For this review, take the finished solid that the model builds, in its own axes (mm). A direction names the side the tool comes from. Coordinates: 2 decimals unless noted, no trailing zeros. Order: outer loops, then holes, each group sorted by start corner. A loop starts at its lowest first (then second) coordinate and runs counter-clockwise, first axis right, second up. Notation, with made-up numbers: M 43,23.5 L 47,23.5 A18 ccw 47,35.5 Z; hole C 4,81 d5. An arc over 180 degrees is marked long. Use one line per item in the form item = value. Start each with the question number.
```python
from build123d import *

# Parameters (mm, degrees)
SKETCH_1_W          = 28
SKETCH_1_H          = 16
EXTRUDE_1_DEPTH     = 5.25
FILLET_1_R          = 3
CUT_EXTRUDE_1_REACH = 21.242
SKETCH_2_R          = 1.5
SKETCH_3_W          = 8.6
SKETCH_3_H          = 6.2
EXTRUDE_2_DEPTH     = 3.4
CUT_EXTRUDE_2_REACH = 21.892
SKETCH_4_W          = 7.6
SKETCH_4_H          = 2.4
SKETCH_5_W          = 8.88
SKETCH_5_H          = 1
EXTRUDE_3_DEPTH     = 3
SKETCH_6_W          = 2.8
SKETCH_6_H          = 4.2
EXTRUDE_4_DEPTH     = 3
FILLET_2_R          = 1.2
EXTRUDE_2_2_DEPTH   = 1.5
SKETCH_7_3_R        = 2.4
EXTRUDE_5_DEPTH     = 3.55
EXTRUDE_6_DEPTH     = 3.55


with BuildPart() as part:
    # Sketch 1 → Extrude 1 (new, symmetric)
    with BuildSketch(Plane(origin=(0, 0, 0), x_dir=(1, 0, 0), z_dir=(0, 1, 0))):
        Rectangle(SKETCH_1_W, SKETCH_1_H)
    extrude(amount=EXTRUDE_1_DEPTH, both=True)

    # Fillet 1
    fillet_1_edges = [part.edges().sort_by_distance(p)[0] for p in [
        (14, 0, 8),
        (-14, 0, 8),
        (-14, 0, -8),
        (14, 0, -8),
    ]]
    fillet(fillet_1_edges, radius=FILLET_1_R)

    # Sketch 2 → Cut-Extrude 1 (cut, up to next)
    with BuildSketch(Plane(origin=(0, 5.25, 0), x_dir=(1, 0, 0), z_dir=(0, 1, 0)), mode=Mode.PRIVATE) as cut_extrude_1_sk1:
        with Locations(Location((11, 5.25, 0), (0, 0, 270))):
            Circle(SKETCH_2_R)
    cut_extrude_1_tool1 = extrude(cut_extrude_1_sk1.sketch, amount=-CUT_EXTRUDE_1_REACH, mode=Mode.PRIVATE) & part.part
    # Sketch 2 → Cut-Extrude 1 (cut, up to next)
    with BuildSketch(Plane(origin=(0, 5.25, 0), x_dir=(1, 0, 0), z_dir=(0, 1, 0)), mode=Mode.PRIVATE) as cut_extrude_1_sk2:
        with Locations(Location((-11, -5.25, 0), (0, 0, 270))):
            Circle(SKETCH_2_R)
    cut_extrude_1_tool2 = extrude(cut_extrude_1_sk2.sketch, amount=-CUT_EXTRUDE_1_REACH, mode=Mode.PRIVATE) & part.part
    add(cut_extrude_1_tool1.solids().sort_by_distance((11, 5.25, -5.25))[0], mode=Mode.SUBTRACT)
    add(cut_extrude_1_tool2.solids().sort_by_distance((-11, 5.25, 5.25))[0], mode=Mode.SUBTRACT)

    # Sketch 3 → Extrude 2 (add)
    with BuildSketch(Plane.XY.offset(8)):
        with Locations((5.6, 0)):
            Rectangle(SKETCH_3_W, SKETCH_3_H)
    extrude(amount=EXTRUDE_2_DEPTH)

    # Sketch 4 → Cut-Extrude 2 (cut, up to next)
    with BuildSketch(Plane(origin=(0, 3.1, 0), x_dir=(1, 0, 0), z_dir=(0, 1, 0)), mode=Mode.PRIVATE) as cut_extrude_2_sk1:
        with Locations((6.1, -9.2)):
            Rectangle(SKETCH_4_W, SKETCH_4_H)
    cut_extrude_2_tool1 = extrude(cut_extrude_2_sk1.sketch, amount=-CUT_EXTRUDE_2_REACH, mode=Mode.PRIVATE) & part.part
    add(cut_extrude_2_tool1.solids().sort_by_distance((6.1, 3.1, 9.2))[0], mode=Mode.SUBTRACT)

    # Sketch 5 → Extrude 3 (add, symmetric)
    with BuildSketch(Plane(origin=(0, 0, 0), x_dir=(1, 0, 0), z_dir=(0, 1, 0))):
        with Locations((18.44, 2.44)):
            Rectangle(SKETCH_5_W, SKETCH_5_H)
        with Locations((18.44, -2.44)):
            Rectangle(SKETCH_5_W, SKETCH_5_H)
    extrude(amount=EXTRUDE_3_DEPTH, both=True)

    # Sketch 6 → Extrude 4 (add)
    with BuildSketch(Plane(origin=(0, 0, -8), x_dir=(-1, 0, 0), z_dir=(0, 0, -1))):
        with Locations((9.9, 0)):
            Rectangle(SKETCH_6_W, SKETCH_6_H)
    extrude(amount=EXTRUDE_4_DEPTH)

    # Fillet 2
    fillet_2_edges = [part.edges().sort_by_distance(p)[0] for p in [
        (-8.5, 0, -11),
        (-11.3, 0, -11),
    ]]
    fillet(fillet_2_edges, radius=FILLET_2_R)

    # Sketch 7 → Extrude 2 2 (add, symmetric)
    with BuildSketch(Plane(origin=(0, 0, 0), x_dir=(1, 0, 0), z_dir=(0, 1, 0))):
        Polygon((3.1, 8), (3.1, 9.617031783), (-9.450182098, 11.481544235), (-9.597133805, 10.492400568), (2.1, 8.754620871), (2.1, 8), align=None)
    extrude(amount=EXTRUDE_2_2_DEPTH, both=True)



with BuildPart() as body_2:
    # Sketch 7_3 → Extrude 5 (new, symmetric)
    with BuildSketch(Plane(origin=(0, 0, 0), x_dir=(1, 0, 0), z_dir=(0, 1, 0))):
        with Locations(Location((-9.6, 14.1, 0), (0, 0, 270))):
            Circle(SKETCH_7_3_R)
    extrude(amount=EXTRUDE_5_DEPTH, both=True)


with BuildPart() as part_1:
    add(part.part)

    add(body_2.part)  # Extrude 6 merges body 2
    # Sketch 8 → Extrude 6 (add, symmetric)
    with BuildSketch(Plane(origin=(0, 0, 0), x_dir=(1, 0, 0), z_dir=(0, 1, 0))):
        with BuildLine():
            Line((-8.741039597, 14.325013226), (-7.870397769, 11.001444789))
            ThreePointArc((-7.870397769, 11.001444789), (-8.504344946, 9.917471161), (-9.588318574, 10.551418337))
            Line((-9.588318574, 10.551418337), (-10.458960403, 13.874986774))
            ThreePointArc((-10.458960403, 13.874986774), (-9.825013226, 14.958960403), (-8.741039597, 14.325013226))
        make_face()
    extrude(amount=EXTRUDE_6_DEPTH, both=True)


solid = part_1.part
```
1. To check wall thickness, follow line 1 (Z direction, x = -3, y = -4.5); line 2 (Z direction, x = 18, y = 1.5); line 3 (Z direction, x = -4.5, y = 0.75). State the ranges of each line that lie inside material, in increasing order.
2. Consider section D-D, the plane y = 0. Give the number of separate pieces and of enclosed holes in the cut face, plus the area to 3 significant figures.
3. Consider section A-A, the plane z = 5.75. Write out the cut boundary in (x, y), plus the area to 3 significant figures.
4. The part is to be moulded in two halves that separate along X. For faces 5 (the flat face through (5, -3.1, 11)), 6 (the flat face through (2.3, 0, 9)), 7 (the cylindrical face through (11.07, 0.07, -6.75)), say which applies: pulls with the +X half, pulls with the -X half, needs draft (parallel to the pull), parting line crosses it, or undercut.
5. Consider section C-C, the plane z = 9.75. Write out the cut boundary in (x, y).
6. Consider section B-B, the plane x = -5. Write out the cut boundary in (y, z), plus the area to 3 significant figures.
7. For pin 1 Ø2.5 at (x, z) = (3.5, 9.5) entering from -Y; pin 2 Ø0.7 at (y, z) = (1, 9.5) entering from +X; pin 3 Ø0.8 at (y, z) = (0, 11) entering from +X, all flat-tipped, find the tip position at first contact; note any pin that passes through.
8. Tool access review of faces 1 (the flat face through (-10, 3.55, -14)), 2 (the cylindrical face through (-8.208, 0.05, -10.058)), 3 (the flat face through (1.3, 0, 10)), 4 (the flat face through (5, 3.1, 11)): name each direction out of +Z, -Z, +X, -X, +Y, -Y from which nothing blocks a thin tool from reaching the whole face with its end or side.
Answers follow:
q1.line_1 = -8 to 8
q1.line_2 = -2.94 to -1.94, 1.94 to 2.94
q1.line_3 = -10.75 to -9.74, -8 to 8
q2.separate_pieces = 1
q2.enclosed_holes = 3
q2.area = 495 mm²
q3.outline = M -13.9,-5.25 L -12.41,-5.25 L -12.41,5.25 L -13.9,5.25 Z; M -9.59,-5.25 L 13.9,-5.25 L 13.9,5.25 L -9.59,5.25 Z
q3.area = 262 mm²
q4.face_5 = needs draft
q4.face_6 = pulls with the +X half
q4.face_7 = undercut
q5.outline = M 1.3,-3.1 L 2.3,-3.1 L 2.3,3.1 L 1.3,3.1 Z
q6.outline = M -5.25,-8 L 5.25,-8 L 5.25,8 L -5.25,8 Z; M -1.5,-10.82 L 1.5,-10.82 L 1.5,-9.81 L -1.5,-9.81 Z
q6.area = 171 mm²
q7.pin_1 = -3.1
q7.pin_2 = 2.3
q7.pin_3 = 9.9
q8.face_1 = -Z, +X, -X, +Y
q8.face_2 = none
q8.face_3 = +Z, -X, +Y, -Y
q8.face_4 = +Z, +X, -X, +Y
